The listing builds one solid part. Answer for the finished solid, in the listing's coordinates (mm). Coordinates: 2 decimals unless noted, no trailing zeros. Order: outer loops, then holes, each group sorted by start corner. A loop starts at its lowest first (then second) coordinate and runs counter-clockwise, first axis right, second up. Notation, with made-up numbers: (-21, 56.25) -> (28, 56.25) arc R19 cw to (28, 63.25) -> close; hole circle Ø10 at (63.5, 59). An arc over 180 degrees is marked (long way). Put each result on its own line as item: value. Start each with the question number.
```python
from build123d import *

# Parameters (mm, degrees)
CROQUIS1_R                    = 12.5
SALIENTE_EXTRUIR1_DEPTH       = 3
TALADRO_DE_MARGEN_PARA_M42_D  = 4.5
TALADRO_DE_MARGEN_PARA_M101_D = 11


with BuildPart() as part:
    # Croquis1 → Saliente-Extruir1 (new body)
    with BuildSketch(Plane.XY):
        with BuildLine():
            Line((70, 25), (0, 25))
            ThreePointArc((0, 25), (-25, 0), (0, -25))
            Line((0, -25), (70, -25))
            ThreePointArc((70, -25), (95, 0), (70, 25))
        make_face()
        with Locations((70, 0)):
            Circle(CROQUIS1_R, mode=Mode.SUBTRACT)
    extrude(amount=SALIENTE_EXTRUIR1_DEPTH)

    # Taladro de margen para M42 (through all)
    with Locations(Plane.XY.offset(3)):
        with Locations((-21, 0), (91, 0), (-10.5, 18.186533479), (10.5, 18.186533479), (21, 0), (10.5, -18.186533479), (-10.5, -18.186533479), (80.5, -18.186533479), (59.5, -18.186533479), (49, 0), (59.5, 18.186533479), (80.5, 18.186533479)):
            Hole(TALADRO_DE_MARGEN_PARA_M42_D / 2)

    # Taladro de margen para M101 (through all)
    with Locations(Plane.XY.offset(3)):
        with Locations((0, 0)):
            Hole(TALADRO_DE_MARGEN_PARA_M101_D / 2)


solid = part.part
```
(1) The part is cut by section D-D on y = -21.5. Determine the outline of the cut face in (x, z), plus the area to 3 significant figures.
(2) For a pull along X with two mould halves and no side action, classify faces 1 (the cylindrical face through (10.99, 15.99, 1.48)), 2 (the flat face through (34, 0, 0)), 3 (the cylindrical face through (94.994, -0.55, 1.479)) as released by +X, released by -X, zero draft, split by the parting line, or undercut.
(3) The part is cut by section B-B on y = -11. Determine the outline of the cut face in (x, z).
(4) The part is cut by section C-C on z = 2.3. Count the separate pieces of the cut face and the enclosed holes in it, plus the area to 3 significant figures.
(5) The part is cut by section A-A on x = 49. Determine the outline of the cut face in (y, z), plus the area to 4 significant figures.
(6) Find the intervals of material crossed by L1, parallel to Y at x = 59.5, z = 1.6; L2, parallel to Y at x = -10.5, z = 1.8; L3, parallel to X at y = 4, z = 2.85, in increasing order.
Worked out:
1. outline: (-12.76, 0) -> (82.76, 0) -> (82.76, 3) -> (-12.76, 3) -> close
1. area: 287 mm2
2. face 1: undercut
2. face 2: zero draft
2. face 3: released by +X
3. outline: (-22.45, 0) -> (64.06, 0) -> (64.06, 3) -> (-22.45, 3) -> close; (75.94, 0) -> (92.45, 0) -> (92.45, 3) -> (75.94, 3) -> close
4. separate pieces: 1
4. enclosed holes: 14
4. area: 4,690 mm2
5. outline: (-25, 0) -> (-2.25, 0) -> (-2.25, 3) -> (-25, 3) -> close; (2.25, 0) -> (25, 0) -> (25, 3) -> (2.25, 3) -> close
5. area: 136.5 mm2
6. L1: -25 to -20.44, -15.94 to -6.78, 6.78 to 15.94, 20.44 to 25
6. L2: -22.69 to -20.44, -15.94 to 15.94, 20.44 to 22.69
6. L3: -24.68 to -3.77, 3.77 to 58.16, 81.84 to 94.68
